For this review, take the finished solid that the model builds, in its own axes (mm). Face numbers are marked on the shaded views. A direction names the side the tool comes from. Give positions to 0.01 mm unless a question says otherwise; leave off trailing zeros. Order: outer loops, then holes, each group sorted by start corner. A loop starts at its lowest first (then second) coordinate and runs counter-clockwise, first axis right, second up. Notation, with made-up numbers: (21.25, -37) - (62.25, -37) arc R19 ccw to (62.25, -16) - close; hole circle Ø6 at (53, 47.25). An arc over 180 degrees is marked (long way). Put each result on its own line as item: value. Start each with the question number.
```python
from build123d import *

# Parameters (mm, degrees)
SKETCH1_R           = 22
BOSS_EXTRUDE1_DEPTH = 7
SKETCH2_W           = 41.36423576
SKETCH2_H           = 15
BOSS_EXTRUDE2_DEPTH = 23
BOSS_EXTRUDE3_DEPTH = 7
SKETCH4_W           = 41.36423576
SKETCH4_H           = 23
BOSS_EXTRUDE4_DEPTH = 3
SKETCH5_R           = 1.5
CUT_EXTRUDE1_DEPTH  = 61.728905803
SKETCH6_R           = 22
CUT_EXTRUDE2_DEPTH  = 46.387222977


with BuildPart() as part:
    # Sketch1 → Boss-Extrude1 (new body)
    with BuildSketch(Plane.XY):
        Circle(SKETCH1_R)
    extrude(amount=BOSS_EXTRUDE1_DEPTH)

    # Sketch2 → Boss-Extrude2 (add)
    with BuildSketch(Plane.XY.offset(7)):
        Rectangle(SKETCH2_W, SKETCH2_H)
    extrude(amount=BOSS_EXTRUDE2_DEPTH)


with BuildPart() as body_2:
    # Sketch3 → Boss-Extrude3 (new body)
    with BuildSketch(Plane(origin=(0, 0, 0), x_dir=(-1, 0, 0), z_dir=(0, 0, -1))):
        with BuildLine():
            Line((-20.68211788, 7.5), (-20.68211788, 26))
            Line((-20.68211788, 26), (20.68211788, 26))
            Line((20.68211788, 26), (20.68211788, 7.5))
            ThreePointArc((20.68211788, 7.5), (0, 22), (-20.68211788, 7.5))
        make_face()
    extrude(amount=-BOSS_EXTRUDE3_DEPTH)

    # Sketch4 → Boss-Extrude4 (add)
    with BuildSketch(Plane(origin=(0, 26, 0), x_dir=(1, 0, 0), z_dir=(0, 1, 0))):
        with Locations((0, -18.5)):
            Rectangle(SKETCH4_W, SKETCH4_H)
    extrude(amount=-BOSS_EXTRUDE4_DEPTH)


with BuildPart() as cut_extrude1_tool:
    # Sketch5 → Cut-Extrude1 (new, through all)
    with BuildSketch(Plane(origin=(0, 26, 0), x_dir=(1, 0, 0), z_dir=(0, 1, 0))):
        with Locations(Location((-10, -3.5, 0), (0, 0, 270))):
            Circle(SKETCH5_R)
        with Locations(Location((10, -3.5, 0), (0, 0, 270))):
            Circle(SKETCH5_R)
    extrude(amount=-CUT_EXTRUDE1_DEPTH)


with BuildPart() as part_1:
    add(part.part)

    # Cut-Extrude1: cut by cut_extrude1_tool
    add(cut_extrude1_tool.part, mode=Mode.SUBTRACT)

    # Sketch6 → Cut-Extrude2 (cut, through all)
    with BuildSketch(Plane(origin=(0, 0, 0), x_dir=(-1, 0, 0), z_dir=(0, 0, -1))):
        Circle(SKETCH6_R)
    extrude(amount=-CUT_EXTRUDE2_DEPTH, mode=Mode.SUBTRACT)


with BuildPart() as body_2_1:
    add(body_2.part)

    # Cut-Extrude1: cut by cut_extrude1_tool
    add(cut_extrude1_tool.part, mode=Mode.SUBTRACT)


solid = body_2_1.part
```
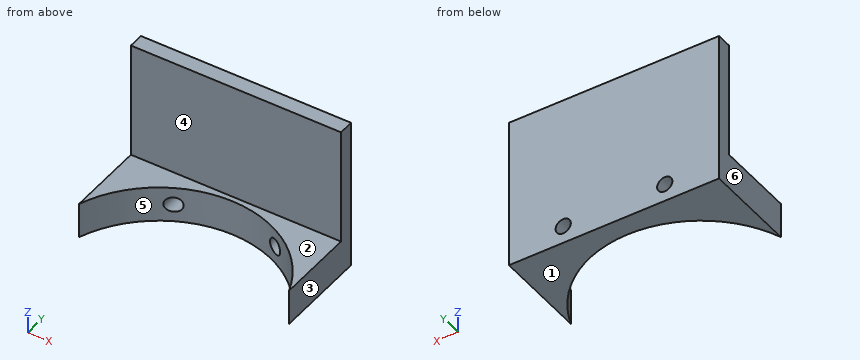
1. Clearance check with flat-ended pins moving along their axes: pin 1 (10 mm diameter, centred on x = -4.5, y = 16, fed in from +Z); pin 2 (1.5 mm diameter, centred on x = -15.5, y = 20, fed in from +Z); pin 3 (5 mm diameter, centred on x = -10, z = 3.5, fed in from +Y). State where each tip first meets the part, or that it passes through.
2. Tool access review of the marked faces 1 and 2: name each direction out of +Z, -Z, +X, -X, +Y, -Y from which nothing blocks a thin tool from reaching the whole face with its end or side.
3. Add section D-D, the plane x = 3.5. Give the boundary of the cut face in (y, z).
4. The part is to be moulded in two halves that separate along X. For the marked faces 3, 4, 5 and 6, say which applies: released by +X, released by -X, zero draft, split by the parting line, or undercut.
5. Add section C-C, the plane x = -10. Give the boundary of the cut face in (y, z), then the cut area to 3 significant figures.
6. Add section B-B, the plane z = 3.5. Give the boundary of the cut face in (x, y) (3 decimals).
7. Add section A-A, the plane y = 17.75. Give the boundary of the cut face in (x, z), then the cut area to 3 significant figures.
8. Wall thickness on line 1 (X direction, y = 23, z = 3.5); line 2 (Z direction, x = 10, y = 21.25); line 3 (Z direction, x = 10, y = 23.5): over which ranges is each line inside the solid? List them lowest first. Write a range as from..to.
Found:
1. pin 1: passes through
1. pin 2: stops at z = 7
1. pin 3: stops at y = 26
2. face 1: -Z, +X, -X, +Y, -Y
2. face 2: +Z, +X, -X, -Y
3. outline: (21.72, 0) - (26, 0) - (26, 30) - (23, 30) - (23, 7) - (21.72, 7) - close
4. face 3: released by +X
4. face 4: zero draft
4. face 5: undercut
4. face 6: released by -X
5. outline: (19.6, 0) - (26, 0) - (26, 2) - (19.6, 2) - close; (19.6, 5) - (26, 5) - (26, 30) - (23, 30) - (23, 7) - (19.6, 7) - close
5. area: 94.6 mm^2
6. outline: (-20.682, 7.5) arc R22 cw to (-11.5, 18.755) - (-11.5, 26) - (-20.682, 26) - close; (-8.5, 20.292) arc R22 cw to (8.5, 20.292) - (8.5, 26) - (-8.5, 26) - close; (11.5, 18.755) arc R22 cw to (20.682, 7.5) - (20.682, 26) - (11.5, 26) - close
7. outline: (-20.68, 0) - (-13, 0) - (-13, 7) - (-20.68, 7) - close; (13, 0) - (20.68, 0) - (20.68, 7) - (13, 7) - close
7. area: 108 mm^2
8. line 1: x = -20.68..-11.5, -8.5..8.5, 11.5..20.68
8. line 2: z = 0..2, 5..7
8. line 3: z = 0..2, 5..30
